from build123d import *

# Parameters (mm, degrees)
IZIM1_R                     = 2.5
Y_KSEKLIK_EKSTR_ZYON1_DEPTH = 7
Y_KSEKLIK_EKSTR_ZYON2_DEPTH = 3
IZIM4_R                     = 19
Y_KSEKLIK_EKSTR_ZYON4_DEPTH = 1.2
RADYUS1_R                   = 0.5
IZIM6_R                     = 5
KES_EKSTR_ZYON2_DEPTH       = 12.2


with BuildPart() as part:
    # Çizim1 → Yükseklik-Ekstrüzyon1 (new body)
    with BuildSketch(Plane.XY):
        with BuildLine():
            Line((-28.709869289, 29.893846154), (21.290130711, 29.893846154))
            ThreePointArc((21.290130711, 29.893846154), (24.825664617, 28.42938006), (26.290130711, 24.893846154))
            Line((26.290130711, 24.893846154), (26.290130711, -25.106153846))
            ThreePointArc((26.290130711, -25.106153846), (24.825664617, -28.641687752), (21.290130711, -30.106153846))
            Line((21.290130711, -30.106153846), (-28.709869289, -30.106153846))
            ThreePointArc((-28.709869289, -30.106153846), (-32.245403195, -28.641687752), (-33.709869289, -25.106153846))
            Line((-33.709869289, -25.106153846), (-33.709869289, 24.893846154))
            ThreePointArc((-33.709869289, 24.893846154), (-32.245403195, 28.42938006), (-28.709869289, 29.893846154))
        make_face()
        with Locations((-28.709869289, 24.893846154)):
            Circle(IZIM1_R, mode=Mode.SUBTRACT)
        with Locations((21.290130711, 24.893846154)):
            Circle(IZIM1_R, mode=Mode.SUBTRACT)
        with Locations((21.290130711, -25.106153846)):
            Circle(IZIM1_R, mode=Mode.SUBTRACT)
        with Locations((-28.709869289, -25.106153846)):
            Circle(IZIM1_R, mode=Mode.SUBTRACT)
    extrude(amount=Y_KSEKLIK_EKSTR_ZYON1_DEPTH)

    # Çizim2 → Yükseklik-Ekstrüzyon2 (add)
    with BuildSketch(Plane.XY.offset(7)):
        with BuildLine():
            Line((13.290130711, 29.893846154), (-20.709869289, 29.893846154))
            ThreePointArc((-20.709869289, 29.893846154), (-22.831189632, 29.015166497), (-23.709869289, 26.893846154))
            Line((-23.709869289, 26.893846154), (-23.709869289, 24.893846154))
            ThreePointArc((-23.709869289, 24.893846154), (-25.174335383, 21.358312248), (-28.709869289, 19.893846154))
            Line((-28.709869289, 19.893846154), (-30.709869289, 19.893846154))
            ThreePointArc((-30.709869289, 19.893846154), (-32.831189632, 19.015166497), (-33.709869289, 16.893846154))
            Line((-33.709869289, 16.893846154), (-33.709869289, -17.106153846))
            ThreePointArc((-33.709869289, -17.106153846), (-32.831189632, -19.22747419), (-30.709869289, -20.106153846))
            Line((-30.709869289, -20.106153846), (-28.709869289, -20.106153846))
            ThreePointArc((-28.709869289, -20.106153846), (-25.174335383, -21.57061994), (-23.709869289, -25.106153846))
            Line((-23.709869289, -25.106153846), (-23.709869289, -27.106153846))
            ThreePointArc((-23.709869289, -27.106153846), (-22.831189632, -29.22747419), (-20.709869289, -30.106153846))
            Line((-20.709869289, -30.106153846), (13.290130711, -30.106153846))
            ThreePointArc((13.290130711, -30.106153846), (15.411451055, -29.22747419), (16.290130711, -27.106153846))
            Line((16.290130711, -27.106153846), (16.290130711, -25.106153846))
            ThreePointArc((16.290130711, -25.106153846), (17.754596805, -21.57061994), (21.290130711, -20.106153846))
            Line((21.290130711, -20.106153846), (23.290130711, -20.106153846))
            ThreePointArc((23.290130711, -20.106153846), (25.411451055, -19.22747419), (26.290130711, -17.106153846))
            Line((26.290130711, -17.106153846), (26.290130711, 16.893846154))
            ThreePointArc((26.290130711, 16.893846154), (25.411451055, 19.015166497), (23.290130711, 19.893846154))
            Line((23.290130711, 19.893846154), (21.290130711, 19.893846154))
            ThreePointArc((21.290130711, 19.893846154), (17.754596805, 21.358312248), (16.290130711, 24.893846154))
            Line((16.290130711, 24.893846154), (16.290130711, 26.893846154))
            ThreePointArc((16.290130711, 26.893846154), (15.411451055, 29.015166497), (13.290130711, 29.893846154))
        make_face()
    extrude(amount=Y_KSEKLIK_EKSTR_ZYON2_DEPTH)

    # Çizim4 → Yükseklik-Ekstrüzyon4 (add)
    with BuildSketch(Plane(origin=(0, 0, 0), x_dir=(-1, 0, 0), z_dir=(0, 0, -1))):
        with Locations((3.709869289, -0.106153846)):
            Circle(IZIM4_R)
    extrude(amount=Y_KSEKLIK_EKSTR_ZYON4_DEPTH)

    # Radyus1
    radyus1_edges = [part.edges().sort_by_distance(p)[0] for p in [
        (-31.209869289, 24.893846154, 0),
        (18.790130711, 24.893846154, 0),
        (18.790130711, -25.106153846, 0),
        (-31.209869289, -25.106153846, 0),
    ]]
    fillet(radyus1_edges, radius=RADYUS1_R)

    # Çizim6 → Kes-Ekstrüzyon2 (cut, through all)
    with BuildSketch(Plane(origin=(0, 0, -1.2), x_dir=(-1, 0, 0), z_dir=(0, 0, -1))):
        with Locations((3.709869289, -0.106153846)):
            Circle(IZIM6_R)
    extrude(amount=-KES_EKSTR_ZYON2_DEPTH, mode=Mode.SUBTRACT)


solid = part.part
The model under review builds one solid part; all positions refer to its coordinate system, in mm. A direction names the side the tool comes from. Give positions to 0.01 mm unless a question says otherwise; leave off trailing zeros. Order: outer loops, then holes, each group sorted by start corner. A loop starts at its lowest first (then second) coordinate and runs counter-clockwise, first axis right, second up. Notation, with made-up numbers: M 83.25,0.25 L 113.25,0.25 A14 ccw 113.25,14.25 Z; hole C 27.25,48 d9. An arc over 180 degrees is marked long. Answer in a Markdown table with one row per item. Add a question column.
1. For pin 1 Ø1 at (y, z) = (26, 8) entering from +X; pin 2 Ø1.6 at (x, z) = (22.5, 8.5) entering from -Y; pin 3 Ø6.5 at (x, y) = (21.29, 24.89) entering from -Z; pin 4 Ø4 at (x, y) = (-28.71, -25.11) entering from +Z, all flat-tipped, find the tip position at first contact; note any pin that passes through.
2. Add section A-A on x = -7. State the section outline as (y, z) points.
3. Mouldability with a two-part tool opening along X and no side actions: class faces 1 (the flat face through (-26, 25, 7)), 2 (the cylindrical face through (17.794, 21.32, 8.479)), 3 (the cylindrical face through (-27.556, -27.324, 3.704)), 4 (the cylindrical face through (-32.854, -19.204, 8.479)) as released by +X, released by -X, zero draft, split by the parting line, or undercut.
4. Add section D-D on x = -25. State the section outline as (y, z) points, plus the area to 3 significant figures.
5. Machinability: for faces 5 (the cylindrical face through (15.435, 28.992, 8.479)), 6 (the flat face through (-23.71, -26, 8)), 7 (the flat face through (22, -20.106, 8)), 8 (the cylindrical face through (-25.136, 21.397, 8.479)), which of the approach directions +Z, -Z, +X, -X, +Y, -Y give a long, thin tool a straight path to every point of the face, cutting with its end or side? Answer none if there is none.
6. Add section B-B on y = 3.5. State the section outline as (x, z) points, plus the area to 3 significant figures.
7. Add section C-C on z = 9. State the section outline as (x, y) points, plus the area to 3 significant figures.
8. To check wall thickness, follow line 1 along Y through (x, z) = (21.5, 4); line 2 along Y through (x, z) = (19, 2.5); line 3 along X through (y, z) = (0, 1.25). State the ranges of each line that lie inside material, in increasing order.
The answers:
| question | item | result |
|---|---|---|
| 1 | pin 1 | x = 16.29 |
| 1 | pin 2 | y = -20.11 |
| 1 | pin 3 | z = 0 |
| 1 | pin 4 | through |
| 2 | outline | M -30.11,0 L -18.82,0 L -18.82,-1.2 L -3.87,-1.2 L -3.87,10 L -30.11,10 Z; M 3.66,-1.2 L 18.61,-1.2 L 18.61,0 L 29.89,0 L 29.89,10 L 3.66,10 Z |
| 3 | face 1 | zero draft |
| 3 | face 2 | released by +X |
| 3 | face 3 | undercut |
| 3 | face 4 | released by -X |
| 4 | outline | M -30.11,0 L 29.89,0 L 29.89,7 L 21.54,7 L 21.54,10 L -21.75,10 L -21.75,7 L -30.11,7 Z |
| 4 | area | 550 mm2 |
| 5 | face 5 | +Z, +X, +Y |
| 5 | face 6 | +Z, -X, -Y |
| 5 | face 7 | +Z, +X, -Y |
| 5 | face 8 | +Z, -X, +Y |
| 6 | outline | M -33.71,0 L -22.36,0 L -22.36,-1.2 L -7.17,-1.2 L -7.17,10 L -33.71,10 Z; M -0.25,-1.2 L 14.94,-1.2 L 14.94,0 L 26.29,0 L 26.29,10 L -0.25,10 Z |
| 6 | area | 567 mm2 |
| 7 | outline | M -33.71,-17.11 A3 ccw -30.71,-20.11 L -28.71,-20.11 A5 cw -23.71,-25.11 L -23.71,-27.11 A3 ccw -20.71,-30.11 L 13.29,-30.11 A3 ccw 16.29,-27.11 L 16.29,-25.11 A5 cw 21.29,-20.11 L 23.29,-20.11 A3 ccw 26.29,-17.11 L 26.29,16.89 A3 ccw 23.29,19.89 L 21.29,19.89 A5 cw 16.29,24.89 L 16.29,26.89 A3 ccw 13.29,29.89 L -20.71,29.89 A3 ccw -23.71,26.89 L -23.71,24.89 A5 cw -28.71,19.89 L -30.71,19.89 A3 ccw -33.71,16.89 Z; hole C -3.71,-0.11 d10 |
| 7 | area | 3,130 mm2 |
| 8 | line 1 | -30.1 to -27.6, -22.61 to 22.4, 27.39 to 29.89 |
| 8 | line 2 | -30.11 to -26.11, -24.1 to 23.89, 25.9 to 29.89 |
| 8 | line 3 | -33.71 to -8.71, 1.29 to 26.29 |
